Input: part model. Units: mm. Frame: model coordinates. A direction names the side the tool comes from. Coordinates: 2 decimals unless noted, no trailing zeros. Loops run counter-clockwise (first coordinate to the right, second up) from the corner with the lowest first, then second, coordinate; pieces in that order, holes last. Notation, with made-up numbers: (61.5, 66) -> (116.5, 66) arc R15 ccw to (116.5, 90) -> close; hole circle Ø7 at (74.5, -32.5). An arc over 180 degrees is marked (long way). Put each result on its own line as item: value. Start each with the question number.
1) Cut plane C-C (z = 16.5). Return the cut outline in (x, y).
2) Cut plane D-D (y = -3). Return the cut outline in (x, z), plus the area to 3 significant figures.
3) Contact query for flat-ended pins moving along their axis: P1, Ø4, axis at x = -8.5, z = 3.5, coming from the +Y side; P2, Ø4, axis at x = -14, y = -0.5, coming from the +Z side; P3, Ø2, axis at y = -13.5, z = 3, coming from the +X side. Output: stop coordinate, or through.
4) Material intervals for L1, parallel to Z at x = -5, y = 8.5; L2, parallel to X at y = 4.5, z = 0.5; L3, parallel to Y at x = -25.5, z = 10, sorted ascending.
5) Cut plane A-A (y = -20). Return the cut outline in (x, z), plus the area to 3 significant figures.
6) Set-up query: faces 1 (the flat face through (-10, -10, -20)), 2 (the flat face through (-20, 0, 15)), 3 (the flat face through (-10, -15, 15)). Return all of +Z, -Z, +X, -X, +Y, -Y with unobstructed straight access to the full face (end or side cutting, diameter ignored); none if empty.
7) Cut plane B-B (x = -2.5). Return the cut outline in (y, z).
from build123d import *

# Parameters (mm, degrees)
SKETCH1_W           = 20
SKETCH1_H           = 30
BOSS_EXTRUDE1_DEPTH = 30
SKETCH2_W           = 40
SKETCH2_H           = 40
BOSS_EXTRUDE2_DEPTH = 20
FILLET1_R           = 10


with BuildPart() as part:
    # Sketch1 → Boss-Extrude1 (new body)
    with BuildSketch(Plane.XY):
        with Locations((-20, -15)):
            Rectangle(SKETCH1_W, SKETCH1_H)
    extrude(amount=BOSS_EXTRUDE1_DEPTH)

    # Sketch2 → Boss-Extrude2 (add)
    with BuildSketch(Plane.XY):
        with Locations((-10, -10)):
            Rectangle(SKETCH2_W, SKETCH2_H)
    extrude(amount=-BOSS_EXTRUDE2_DEPTH)

    # Fillet1
    fillet1_edges = [part.edges().sort_by_distance(p)[0] for p in [
        (-20, 0, 0),
        (10, 10, -10),
        (-20, 0, 30),
    ]]
    fillet(fillet1_edges, radius=FILLET1_R - 0.0001)  # a hair under: the kernel refuses the full size


solid = part.part
Results found:
1. outline: (-30, -30) -> (-10, -30) -> (-10, 0) -> (-30, 0) -> close
2. outline: (-30, -20) -> (10, -20) -> (10, 0) -> (-10, 0) -> (-10, 27.14) -> (-30, 27.14) -> close
2. area: 1,340 mm2
3. P1: stops at y = 3.77
3. P2: stops at z = 26.61
3. P3: stops at x = -10
4. L1: z = -20 to 0
4. L2: x = -30 to -10
4. L3: y = -30 to 0
5. outline: (-30, -20) -> (10, -20) -> (10, 0) -> (-10, 0) -> (-10, 30) -> (-30, 30) -> close
5. area: 1,400 mm2
6. face 1: -Z, +X, -X, +Y, -Y
6. face 2: +Z, +X, -X, +Y
6. face 3: +Z, +X, +Y, -Y
7. outline: (-30, -20) -> (10, -20) -> (10, 0) -> (-30, 0) -> close
